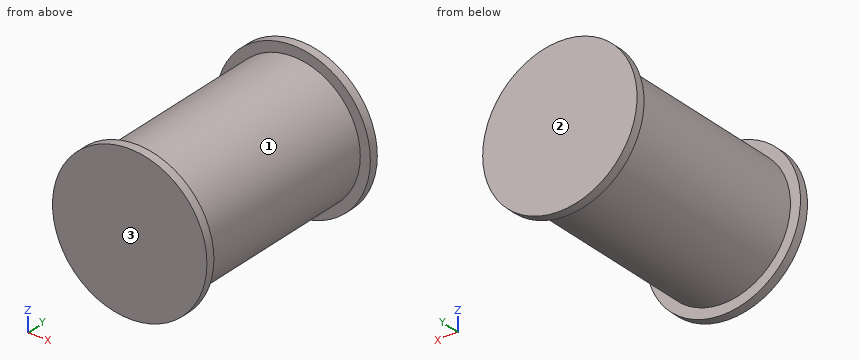
```python
from build123d import *

# Parameters (mm, degrees)
F0_R          = 1.9020393282
F1_DEPTH      = 2.8448
F1_DEPTH_BACK = 2.8448
F2_R          = 2.1870906788
F3_DEPTH      = 0.254


# Not quite as in the source:
# - a pattern or mirror of a feature is missing from the dataset's text; its kind, count and spacing are read off the source's solid


with BuildPart() as f1:
    # F0 (on Front) → F1 (new body, two sides)
    with BuildSketch(Plane.XZ) as f1_sk:
        Circle(F0_R)
    extrude(amount=F1_DEPTH)
    extrude(f1_sk.sketch, amount=-F1_DEPTH_BACK)

    # F2 (on face) → F3 (join)
    with BuildSketch(Plane.XZ.offset(2.8448)):
        Circle(F2_R)
    f3 = extrude(amount=F3_DEPTH)

    # F3_copies: F3 across plane
    add(f3.mirror(Plane.ZX))


solid = f1.part
```
Model file for the job. Use its own axes, mm. Face numbers are marked on the shaded views. Give positions to 0.01 mm unless a question says otherwise; leave off trailing zeros. Loops run counter-clockwise (first coordinate to the right, second up) from the corner with the lowest first, then second, coordinate; pieces in that order, holes last. Notation, with made-up numbers: (2, 59.25) -> (35, 59.25) arc R22 cw to (35, 80.25) -> close; hole circle Ø8 at (9, 17). An arc over 180 degrees is marked (long way). Use CSV: the item, a comma, the result in double quotes. Start each with the question number.
1) Mould opens along Y. For the marked faces 1, 2 and 3 say: released by +Y, released by -Y, zero draft, split by the parting line, or undercut.
2) Slice it at B-B on z = 0. Give the cut face in (x, y).
3) Slice it at A-A on x = 0. Give the cut face in (y, z).
4) Wall check: line 1 (Z direction, x = 0.55, y = -1); line 2 (X direction, y = 1, z = -1.45); line 3 (Z direction, x = 0.75, y = 0). Give the ranges that are in metal, low to high.
5) Slice it at C-C on y = -1.75. Give the cut face in (x, z).
Computed values:
1,face 1,"undercut"
1,face 2,"released by +Y"
1,face 3,"released by -Y"
2,outline,"(-2.19, -3.1) -> (2.19, -3.1) -> (2.19, -2.84) -> (1.9, -2.84) -> (1.9, 2.84) -> (2.19, 2.84) -> (2.19, 3.1) -> (-2.19, 3.1) -> (-2.19, 2.84) -> (-1.9, 2.84) -> (-1.9, -2.84) -> (-2.19, -2.84) -> close"
3,outline,"(-3.1, -2.19) -> (-2.84, -2.19) -> (-2.84, -1.9) -> (2.84, -1.9) -> (2.84, -2.19) -> (3.1, -2.19) -> (3.1, 2.19) -> (2.84, 2.19) -> (2.84, 1.9) -> (-2.84, 1.9) -> (-2.84, 2.19) -> (-3.1, 2.19) -> close"
4,line 1,"z = -1.82 to 1.82"
4,line 2,"x = -1.23 to 1.23"
4,line 3,"z = -1.75 to 1.75"
5,outline,"circle Ø3.8 at (0, 0)"
